Here's how the part is built. I have some questions about the finished solid (model axes, mm). A direction names the side the tool comes from. Round coordinates to 2 decimals unless told otherwise and drop trailing zeros. Write each loop counter-clockwise with the first axis right and the second up, starting at its lowest first coordinate (ties: lowest second). Pieces come first, ordered by that corner, then holes. Notation, with made-up numbers: (74.25, -14) -> (79.25, -14) arc R19 ccw to (79.25, 23) -> close; hole circle Ø1 at (-33.75, 24.25). An arc over 180 degrees is marked (long way). Answer as CSV lines item,"result".
```python
from build123d import *

# Parameters (mm, degrees)
F1_DEPTH  = 6.17
F3_DEPTH  = 0.55
F2_R      = 2.4
F4_DEPTH  = 0.58
F6_W      = 4
F6_H      = 0.05
F7_DEPTH  = 0.1
F8_R      = 2.5
F8_R_2    = 0.45
F9_DEPTH  = 0.6
F10_DEPTH = 0.6
F11_R     = 1
F12_DEPTH = 0.7361696724


with BuildPart() as f1:
    # F0 (on Front) → F1 (new body)
    with BuildSketch(Plane.XZ):
        with BuildLine():
            Line((-20.505, -57.575), (20.505, -57.575))
            ThreePointArc((20.505, -57.575), (26.706326471, -55.006326471), (29.275, -48.805))
            Line((29.275, -48.805), (29.275, 48.805))
            ThreePointArc((29.275, 48.805), (26.706326471, 55.006326471), (20.505, 57.575))
            Line((20.505, 57.575), (-20.505, 57.575))
            ThreePointArc((-20.505, 57.575), (-26.706326471, 55.006326471), (-29.275, 48.805))
            Line((-29.275, 48.805), (-29.275, -48.805))
            ThreePointArc((-29.275, -48.805), (-26.706326471, -55.006326471), (-20.505, -57.575))
        make_face()
        with BuildLine():
            ThreePointArc((28.675, -48.805), (26.2820624023, -54.5820624023), (20.505, -56.975))
            Line((20.505, -56.975), (-20.505, -56.975))
            ThreePointArc((-20.505, -56.975), (-26.2820624023, -54.5820624023), (-28.675, -48.805))
            Line((-28.675, -48.805), (-28.675, 48.805))
            ThreePointArc((-28.675, 48.805), (-26.2820624023, 54.5820624023), (-20.505, 56.975))
            Line((-20.505, 56.975), (20.505, 56.975))
            ThreePointArc((20.505, 56.975), (26.2820624023, 54.5820624023), (28.675, 48.805))
            Line((28.675, 48.805), (28.675, -48.805))
        make_face(mode=Mode.SUBTRACT)
    extrude(amount=F1_DEPTH)

    # F2 (on face) → F3 (cut)
    with BuildSketch(Plane.YZ.offset(29.275)):
        with BuildLine():
            Line((-2.335, 45.045), (-3.835, 45.045))
            ThreePointArc((-3.835, 45.045), (-4.3653300859, 44.8253300859), (-4.585, 44.295))
            Line((-4.585, 44.295), (-4.585, 39.795))
            ThreePointArc((-4.585, 39.795), (-4.3653300859, 39.2646699141), (-3.835, 39.045))
            Line((-3.835, 39.045), (-2.335, 39.045))
            ThreePointArc((-2.335, 39.045), (-1.8046699141, 39.2646699141), (-1.585, 39.795))
            Line((-1.585, 39.795), (-1.585, 44.295))
            ThreePointArc((-1.585, 44.295), (-1.8046699141, 44.8253300859), (-2.335, 45.045))
        make_face()
    extrude(amount=-F3_DEPTH, mode=Mode.SUBTRACT)

    # F2 (on face) → F4 (join)
    with BuildSketch(Plane.YZ.offset(29.275)):
        with Locations((-3.085, 32.295)):
            Circle(F2_R)
        with Locations((-3.085, 22.015)):
            Circle(F2_R)
    extrude(amount=F4_DEPTH)

    # F5 (on face) + F6 (on face) → F7 (cut)
    with BuildSketch(Plane.YZ.offset(29.855)):
        Polygon((-3.11, 32.27), (-3.11, 30.295), (-3.06, 30.295), (-3.06, 32.27), (-1.085, 32.27), (-1.085, 32.32), (-3.06, 32.32), (-3.06, 34.295), (-3.11, 34.295), (-3.11, 32.32), (-5.085, 32.32), (-5.085, 32.27), align=None)
    with BuildSketch(Plane.YZ.offset(29.855)):
        with Locations((-3.085, 22.015)):
            Rectangle(F6_W, F6_H)
    extrude(amount=-F7_DEPTH, mode=Mode.SUBTRACT)

    # F8 (on face) → F9 (cut)
    with BuildSketch(Plane.XY.offset(57.575)):
        with Locations((17.235, -3.085)):
            Circle(F8_R)
        with Locations((12.495, -3.085)):
            Circle(F8_R_2)
    extrude(amount=-F9_DEPTH, mode=Mode.SUBTRACT)

    # F8 (on face) → F10 (join)
    with BuildSketch(Plane.XY.offset(57.575)):
        with BuildLine():
            ThreePointArc((-19.835, -3.085), (-19.3956601718, -4.1456601718), (-18.335, -4.585))
            Line((-18.335, -4.585), (-11.235, -4.585))
            ThreePointArc((-11.235, -4.585), (-10.1743398282, -4.1456601718), (-9.735, -3.085))
            ThreePointArc((-9.735, -3.085), (-10.1743398282, -2.0243398282), (-11.235, -1.585))
            Line((-11.235, -1.585), (-18.335, -1.585))
            ThreePointArc((-18.335, -1.585), (-19.3956601718, -2.0243398282), (-19.835, -3.085))
        make_face()
    extrude(amount=F10_DEPTH)

    # F11 (on face) → F12 (cut, through all)
    with BuildSketch(Plane(origin=(0, 0, -57.575), x_dir=(1, 0, 0), z_dir=(0, 0, -1))):
        with BuildLine():
            Line((-10.505, 1.285), (10.505, 1.285))
            ThreePointArc((10.505, 1.285), (10.8585533906, 1.4314466094), (11.005, 1.785))
            Line((11.005, 1.785), (11.005, 4.385))
            ThreePointArc((11.005, 4.385), (10.8585533906, 4.7385533906), (10.505, 4.885))
            Line((10.505, 4.885), (-10.505, 4.885))
            ThreePointArc((-10.505, 4.885), (-10.8585533906, 4.7385533906), (-11.005, 4.385))
            Line((-11.005, 4.385), (-11.005, 1.785))
            ThreePointArc((-11.005, 1.785), (-10.8585533906, 1.4314466094), (-10.505, 1.285))
        make_face()
        with Locations((-13.025, 3.085)):
            Circle(F11_R)
        with Locations((13.025, 3.085)):
            Circle(F11_R)
        with BuildLine():
            Line((-20.835, 1.935), (-16.165, 1.935))
            ThreePointArc((-16.165, 1.935), (-15.3518272016, 2.2718272016), (-15.015, 3.085))
            ThreePointArc((-15.015, 3.085), (-15.3518272016, 3.8981727984), (-16.165, 4.235))
            Line((-16.165, 4.235), (-20.835, 4.235))
            ThreePointArc((-20.835, 4.235), (-21.6481727984, 3.8981727984), (-21.985, 3.085))
            ThreePointArc((-21.985, 3.085), (-21.6481727984, 2.2718272016), (-20.835, 1.935))
        make_face()
        with BuildLine():
            Line((16.165, 1.935), (20.835, 1.935))
            ThreePointArc((20.835, 1.935), (21.6481727984, 2.2718272016), (21.985, 3.085))
            ThreePointArc((21.985, 3.085), (21.6481727984, 3.8981727984), (20.835, 4.235))
            Line((20.835, 4.235), (16.165, 4.235))
            ThreePointArc((16.165, 4.235), (15.3518272016, 3.8981727984), (15.015, 3.085))
            ThreePointArc((15.015, 3.085), (15.3518272016, 2.2718272016), (16.165, 1.935))
        make_face()
    extrude(amount=-F12_DEPTH, mode=Mode.SUBTRACT)


solid = f1.part
```
1. Suppose I cut it at C-C on x = -24.5. Please give me the cut outline in (y, z).
Numbers:
outline,"(-6.17, -56.61) -> (0, -56.61) -> (0, -55.93) -> (-6.17, -55.93) -> close; (-6.17, 55.93) -> (0, 55.93) -> (0, 56.61) -> (-6.17, 56.61) -> close"
2. Suppose I cut it at A-A on z = 41.5. Please give me the cut outline in (x, y) (3 decimals), and give its area (3 significant figures).
Numbers:
outline,"(-29.275, -6.17) -> (-28.675, -6.17) -> (-28.675, 0) -> (-29.275, 0) -> close; (28.675, -6.17) -> (29.275, -6.17) -> (29.275, -4.585) -> (28.725, -4.585) -> (28.725, -1.585) -> (29.275, -1.585) -> (29.275, 0) -> (28.675, 0) -> close"
area,"5.75 mm^2"
3. Suppose I cut it at B-B on x = 5.5. Please give me the cut outline in (y, z) (3 decimals), and give its area (3 significant figures).
Numbers:
outline,"(-6.17, -57.575) -> (-4.885, -57.575) -> (-4.885, -56.975) -> (-6.17, -56.975) -> close; (-6.17, 56.975) -> (0, 56.975) -> (0, 57.575) -> (-6.17, 57.575) -> close; (-1.285, -57.575) -> (0, -57.575) -> (0, -56.975) -> (-1.285, -56.975) -> close"
area,"5.24 mm^2"
4. If we mould it in two halves opening along X, with no side actions, what happens to faces 4 (the face through (29.855, -4, 32)), 5 (the face through (0, -3, 56.975)), 6 (the face through (-26.77, -3.04, -54.94))? For each: released by +X, released by -X, zero draft, split by the parting line, or undercut.
Numbers:
face 4,"released by +X"
face 5,"undercut"
face 6,"released by -X"
5. For pin 1 Ø10 at (x, z) = (-23, -13) entering from +Y; pin 2 Ø1.9 at (y, z) = (-2.5, -13.5) entering from +X (3 decimals), each with a flat end and sliding along its axis, tell me the tip position at first contact or that it passes through.
Numbers:
pin 1,"passes through"
pin 2,"stops at x = 29.275"
6. Suppose I cut it at D-D on z = 26.5. Please give me the cut outline in (x, y) (3 decimals), and give its area (3 significant figures).
Numbers:
outline,"(-29.275, -6.17) -> (-28.675, -6.17) -> (-28.675, 0) -> (-29.275, 0) -> close; (28.675, -6.17) -> (29.275, -6.17) -> (29.275, 0) -> (28.675, 0) -> close"
area,"7.40 mm^2"
7. On a 3-axis mill with a long thin cutter (end or side, diameter ignored), from which of +Z, -Z, +X, -X, +Y, -Y can I reach the whole of each face in a straight line? I mean faces 1 (the face through (14.737, -2.975, 57.279)), 2 (the face through (-12.1, -2.7, -57.3)), 3 (the face through (-28.675, -3, -1)). Say none if no direction works.
Numbers:
face 1,"+Z"
face 2,"-Z"
face 3,"+Y, -Y"
8. If I drill on line 1 (X direction, y = -2.5, z = -14) (3 decimals); line 2 (Z direction, x = 14.5, y = -3.5) (3 decimals); line 3 (Z direction, x = -6, y = -3.75) (3 decimals), over which ranges is the centre line in solid material (lowest first)?
Numbers:
line 1,"x = -29.275 to -28.675, 28.675 to 29.275"
line 2,"z = -57.575 to -56.975, 56.975 to 57.575"
line 3,"z = 56.975 to 57.575"
